Could you check a few things on this model? Use its own coordinates, in mm. Coordinates: 2 decimals unless noted, no trailing zeros. Order: outer loops, then holes, each group sorted by start corner. A loop starts at its lowest first (then second) coordinate and runs counter-clockwise, first axis right, second up. Notation, with made-up numbers: (-3, -38) -> (40, -38) arc R13 cw to (40, -28) -> close; hole circle Ø9 at (3, 26). An arc over 180 degrees is marked (long way). Put each result on its own line as item: value. Start each with the question number.
Q1. If we section it at A-A (z = 26): Count the separate pieces of the cut face and the enclosed holes in it, and give its area (3 significant figures).
Q2. Will these pins go through, and if not, where does the flat tip stop? pin 1 (0.8 mm diameter, centred on y = 1, z = 24.5, fed in from -X); pin 2 (0.5 mm diameter, centred on x = 41.5, y = 0.5, fed in from -Z).
Q3. Please list where these lines run through material, in increasing order: line 1 along X through (y, z) = (0.65, 10.75); line 2 along Z through (x, y) = (14.5, 0.55).
Q4. If we section it at B-B (z = 2.75): Please give me the cut outline in (x, y).
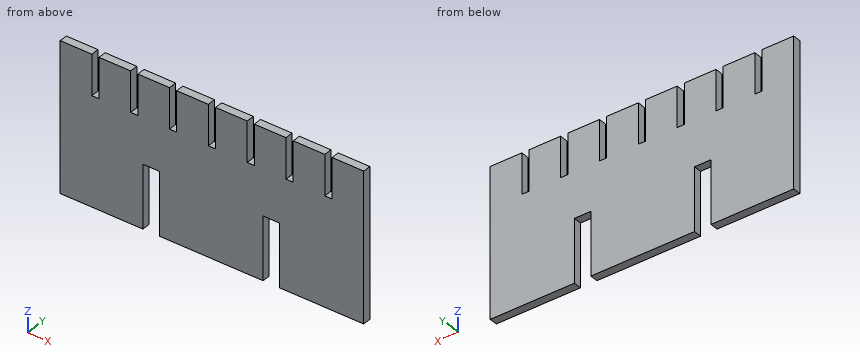
from build123d import *

# Parameters (mm, degrees)
BOSS_EXTRUDE1_DEPTH = 1.6


with BuildPart() as part:
    # Sketch1 → Boss-Extrude1 (new body)
    with BuildSketch(Plane(origin=(0, 0, 0), x_dir=(1, 0, 0), z_dir=(0, 1, 0))):
        Polygon((0, 0), (0, -29.5), (6.25, -29.5), (6.25, -21.5), (7.679, -21.5), (7.679, -29.5), (13.929, -29.5), (13.929, -21.5), (15.358, -21.5), (15.358, -29.5), (21.608, -29.5), (21.608, -21.5), (23.037, -21.5), (23.037, -29.5), (29.287, -29.5), (29.287, -21.5), (30.716, -21.5), (30.716, -29.5), (36.966, -29.5), (36.966, -21.5), (38.395, -21.5), (38.395, -29.5), (44.645, -29.5), (44.645, -21.5), (46.074, -21.5), (46.074, -29.5), (52.324, -29.5), (52.324, -21.5), (53.753, -21.5), (53.753, -29.5), (60.003, -29.5), (60.003, 0), (43.353, 0), (43.353, -12.5), (40.103, -12.5), (40.103, 0), (19.603, 0), (19.603, -12.5), (16.353, -12.5), (16.353, 0), align=None)
    extrude(amount=BOSS_EXTRUDE1_DEPTH)


solid = part.part
The answers:
1. separate pieces: 8
1. enclosed holes: 0
1. area: 80.0 mm^2
2. pin 1: x = 0
2. pin 2: z = 12.5
3. line 1: 0 to 16.35, 19.6 to 40.1, 43.35 to 60
3. line 2: 0 to 21.5
4. outline: (0, 0) -> (16.35, 0) -> (16.35, 1.6) -> (0, 1.6) -> close; (19.6, 0) -> (40.1, 0) -> (40.1, 1.6) -> (19.6, 1.6) -> close; (43.35, 0) -> (60, 0) -> (60, 1.6) -> (43.35, 1.6) -> close
